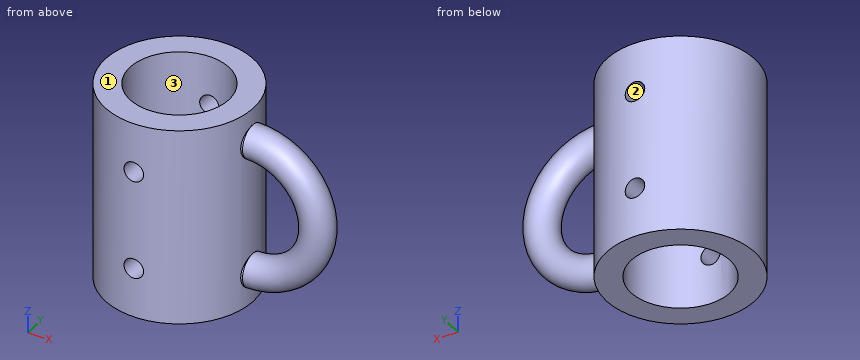
from build123d import *

# Parameters (mm, degrees)
SKETCH1_R                = 22.5
SKETCH1_R_2              = 15
BOSS_EXTRUDE1_DEPTH      = 30
BOSS_EXTRUDE1_DEPTH_BACK = 30
CUT_EXTRUDE1_START       = -50
SKETCH2_R                = 3
CUT_EXTRUDE1_DEPTH       = 80
SKETCH4_R                = 5


with BuildPart() as part:
    # Sketch1 → Boss-Extrude1 (new body, two sides)
    with BuildSketch(Plane.XY) as boss_extrude1_sk:
        Circle(SKETCH1_R)
        Circle(SKETCH1_R_2, mode=Mode.SUBTRACT)
    extrude(amount=BOSS_EXTRUDE1_DEPTH)
    extrude(boss_extrude1_sk.sketch, amount=-BOSS_EXTRUDE1_DEPTH_BACK)

    # Sketch2 → Cut-Extrude1 (cut)
    with BuildSketch(Plane(origin=(0, 0, 0), x_dir=(1, 0, 0), z_dir=(0, 1, 0)).offset(CUT_EXTRUDE1_START)):
        with Locations((0, -15)):
            Circle(SKETCH2_R)
    cut_extrude1 = extrude(amount=CUT_EXTRUDE1_DEPTH, mode=Mode.SUBTRACT)

    # Mirror1: Cut-Extrude1 across plane
    add(cut_extrude1.mirror(Plane.XY), mode=Mode.SUBTRACT)

    # Sweep2: sweep along a path in Sketch3
    with BuildLine(Plane(origin=(0, 0, 0), x_dir=(1, 0, 0), z_dir=(0, 1, 0))) as sweep2_path:
        Line((20, -20), (22.5, -20))
        ThreePointArc((22.5, -20), (42.5, 0), (22.5, 20))
        Line((22.5, 20), (20, 20))
    # Sketch4 → Sweep2 (sweep)
    with BuildSketch(Plane(origin=(20, 0, 0), x_dir=(0, 0, -1), z_dir=(1, 0, 0))):
        with Locations((-20, 0)):
            Circle(SKETCH4_R)
    sweep(path=sweep2_path.line)


solid = part.part
Model file for the job. Use its own axes, mm. Face numbers are marked on the shaded views. Round coordinates to 2 decimals unless told otherwise and drop trailing zeros. Loops run counter-clockwise (first coordinate to the right, second up) from the corner with the lowest first, then second, coordinate; pieces in that order, holes last. Notation, with made-up numbers: (-37, 65.5) -> (21, 65.5) arc R25 cw to (21, 78.5) -> close; hole circle Ø4 at (1, -18). An arc over 180 degrees is marked (long way). Answer as CSV lines item,"result". Start each with the question number.
1) Slice it at C-C (y = 9). List the corners of the cut face in (x, z).
2) Probe line 1 along Z through (x, y) = (0, -19.5); line 2 along X through (y, z) = (3.5, -3.5); line 3 along X through (y, z) = (-6.5, -0.5). List the from-to ranges inside material, lowest first.
3) Mould opens along X. For the marked faces 1, 2 and 3 say: +X half, -X half, draft (parallel to the pull), parting line (faces both ways), or undercut.
4) Pin check, flat tips, straight feed: P1, Ø6, axis at y = -8.5, z = 21.5, coming from the -X side; P2, Ø1, axis at x = 37, y = -1, coming from the +Z side; P3, Ø5.5, axis at x = 0, z = -15, coming from the -Y side; P4, Ø12, axis at x = -8, z = -19.5, coming from the +Y side. Stop position of each tip, or through.
5) Slice it at B-B (x = 0). List the corners of the cut face in (y, z), plus the area to 3 significant figures.
6) Slice it at A-A (y = -1). State how many separate pieces and enclosed holes the cut face has, plus the area to 3 significant figures.
7) Slice it at D-D (y = -18). List the corners of the cut face in (x, z), plus the area to 3 significant figures.
Filled in:
1,outline,"(-20.62, -30) -> (-12, -30) -> (-12, 30) -> (-20.62, 30) -> close; (12, -30) -> (20.62, -30) -> (20.62, 30) -> (12, 30) -> close"
2,line 1,"z = -30 to -18, -12 to 12, 18 to 30"
2,line 2,"x = -22.23 to -14.59, 14.59 to 22.23, 38.55 to 45.81"
2,line 3,"x = -21.54 to -13.52, 13.52 to 21.54"
3,face 1,"draft"
3,face 2,"undercut"
3,face 3,"undercut"
4,P1,"stops at x = -21.82"
4,P2,"stops at z = 20.61"
4,P3,"passes through"
4,P4,"stops at y = 22.41"
5,outline,"(-22.5, -30) -> (-15, -30) -> (-15, -18) -> (-22.5, -18) -> close; (-22.5, -12) -> (-15, -12) -> (-15, 12) -> (-22.5, 12) -> close; (-22.5, 18) -> (-15, 18) -> (-15, 30) -> (-22.5, 30) -> close; (15, -30) -> (22.5, -30) -> (22.5, -18) -> (15, -18) -> close; (15, -12) -> (22.5, -12) -> (22.5, 12) -> (15, 12) -> close; (15, 18) -> (22.5, 18) -> (22.5, 30) -> (15, 30) -> close"
5,area,"720 mm2"
6,separate pieces,"2"
6,enclosed holes,"1"
6,area,"1,520 mm2"
7,outline,"(-13.5, -30) -> (13.5, -30) -> (13.5, 30) -> (-13.5, 30) -> close; hole circle Ø6 at (0, -15); hole circle Ø6 at (0, 15)"
7,area,"1,560 mm2"
